Source: three-view drawing plus pictorial views. Frame: mm from the lowest corner of the part. A direction names the side the tool comes from. Coordinates: 2 decimals unless noted, no trailing zeros. Loops run counter-clockwise (first coordinate to the right, second up) from the corner with the lowest first, then second, coordinate; pieces in that order, holes last.
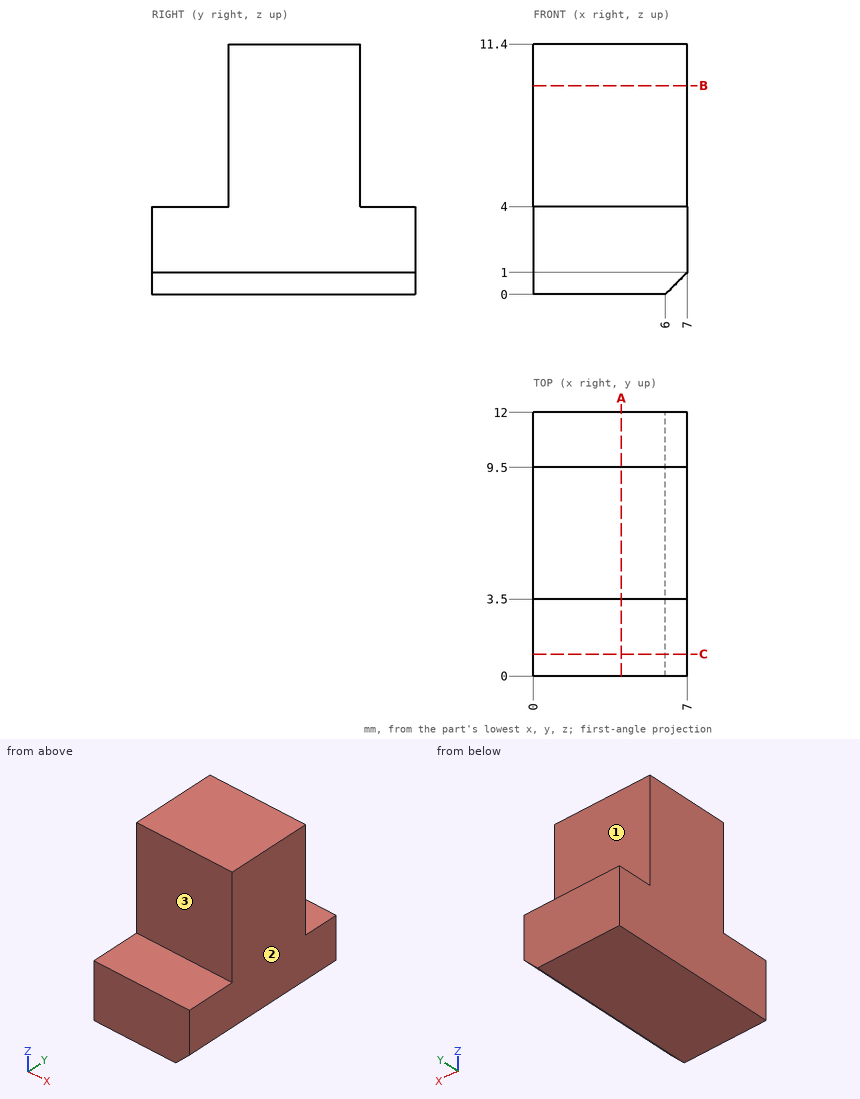
Q1. Contact query for flat-ended pins moving along their axis: pin 1 Ø5 at (y, z) = (7.5, 2.5) entering from -X; pin 2 Ø0.8 at (x, y) = (3.5, 10.5) entering from +Z; pin 3 Ø3.5 at (x, z) = (4, 7) entering from +Y; pin 4 Ø2 at (x, z) = (5, 9) entering from -Y. Output: stop coordinate, or through.
Q2. Section C-C, the plane y = 1. Return the cut outline in (x, z), plus the area to 3 significant figures.
Q3. Line query: line 1 along Y through (x, z) = (5.25, 6.5); line 2 along Z through (x, y) = (4.25, 1); line 3 along Z through (x, y) = (6.25, 5). Output: solid intervals per line, ascending.
Q4. Section A-A, the plane x = 4. Return the cut outline in (y, z), plus the area to 3 significant figures.
Q5. Section B-B, the plane z = 9.5. Return the cut outline in (x, y).
Q6. Access query for the marked faces 1, 2 and 3. Directions: +Z, -Z, +X, -X, +Y, -Y. A direction counts if a zero-diameter tool reaches every point of the face in a straight line with its end or side. Return the directions, or none.
Derived:
1. pin 1: stops at x = 0
1. pin 2: stops at z = 4
1. pin 3: stops at y = 9.5
1. pin 4: stops at y = 3.5
2. outline: (0, 0) - (6, 0) - (7, 1) - (7, 4) - (0, 4) - close
2. area: 27.5 mm2
3. line 1: y = 3.5 to 9.5
3. line 2: z = 0 to 4
3. line 3: z = 0.25 to 11.4
4. outline: (0, 0) - (12, 0) - (12, 4) - (9.5, 4) - (9.5, 11.4) - (3.5, 11.4) - (3.5, 4) - (0, 4) - close
4. area: 92.4 mm2
5. outline: (0, 3.5) - (7, 3.5) - (7, 9.5) - (0, 9.5) - close
6. face 1: +Z, +X, -X, +Y
6. face 2: +Z, -Z, +X, +Y, -Y
6. face 3: +Z, +X, -X, -Y
